Can you work these out from the model? Positions are in its coordinate system, mm. Give positions to 0.01 mm unless a question says otherwise; leave off trailing zeros. Order: outer loops, then holes, each group sorted by start corner. A loop starts at its lowest first (then second) coordinate and runs counter-clockwise, first axis right, second up. Notation, with made-up numbers: M 9,-30.5 L 48,-30.5 A25 ccw 48,-2.5 Z; hole C 28,28 d10. An arc over 180 degrees is marked long. Use a Markdown table: item, result. Add a question column.
Autodesk Inventor part; units mm, degrees
ref_plane "YZ Plane" through (0, 0, 0) normal (1, 0, 0) x (0, 1, 0)
ref_plane "XZ Plane" through (0, 0, 0) normal (0, 1, 0) x (-1, 0, 0)
ref_plane "XY Plane" through (0, 0, 0) normal (0, 0, 1) x (1, 0, 0)
sketch "Sketch1" plane through (0, 0, 0) normal (0, 0, 1) x (1, 0, 0)
  arc A0 (-142.7162, -169.544) -> (-130.9605, -185.7243) centre (-136.8383, -177.6341) ccw
  line L0 (-17.6981, -103.4344) -> (-130.9605, -185.7243)
  line L1 (46.5951, -32.0012) -> (-142.7162, -169.544)
  line L2 (-17.6981, -103.4344) -> (58.3508, -48.1816)
  arc A1 (58.3508, -48.1816) -> (46.5951, -32.0012) centre (52.473, -40.0914) ccw
  circle A2 centre (52.473, -40.0914) radius 4
  circle A3 centre (-136.8383, -177.6341) radius 6
  point P0 (0, 0)
  point P1 (0, 0)
  dimension "d0" = 8
  dimension "d3" = 12
extrude "Extrusion1" add sketch "Sketch1" along normal mid plane 24
properties part number "Second part of arm of gripper"
1. I need wall thicknesses on L1, parallel to Y at x = -131.5, z = -9.25; L2, parallel to Y at x = -93.5, z = 4; L3, parallel to Y at x = 43.5, z = 10. Which ranges of each line are inside material? Lowest first, please. Write a range as [from, to].
2. If we section it at C-C, the plane x = -89: List the corners of the cut face in (y, z) for me.
3. If we section it at B-B, the plane y = -130: List the corners of the cut face in (x, z) for me.
4. If we section it at A-A, the plane z = 5.5: List the corners of the cut face in (x, y) for me.
5. We'd pull the mould along Y, two halves only. Please class faces 1 (the face through (-43, -108, -12)), 2 (the face through (48.477, -40.267, -0.168)), 3 (the face through (-131.296, -175.336, -0.168)), 4 (the face through (-144.797, -183.688, -0.168)): +Y half, -Y half, draft (parallel to the pull), parting line (faces both ways), or undercut.
6. Will these pins go through, and if not, where does the flat tip stop? pin 1 (1.5 mm diameter, centred on y = -123, z = 3.5, fed in from +X); pin 2 (13 mm diameter, centred on x = 52.47, y = -40.09, fed in from +Z); pin 3 (1 mm diameter, centred on x = -25, z = 3, fed in from -Y); pin 4 (2 mm diameter, centred on y = -130, z = -6.5, fed in from +X).
Geometry results:
| question | item | result |
|---|---|---|
| 1 | L1 | y = [-186.09, -180.37], [-174.9, -161.39] |
| 1 | L2 | y = [-158.51, -133.79] |
| 1 | L3 | y = [-58.97, -34.25] |
| 2 | outline | M -155.24,-12 L -130.52,-12 L -130.52,12 L -155.24,12 Z |
| 3 | outline | M -88.29,-12 L -54.26,-12 L -54.26,12 L -88.29,12 Z |
| 4 | outline | M -142.72,-169.54 A10 ccw -130.96,-185.72 L -17.7,-103.43 L 58.35,-48.18 A10 ccw 46.6,-32 Z; hole C -136.84,-177.63 d12; hole C 52.47,-40.09 d8 |
| 5 | face 1 | draft |
| 5 | face 2 | undercut |
| 5 | face 3 | undercut |
| 5 | face 4 | parting line |
| 6 | pin 1 | stops at x = -43.6 |
| 6 | pin 2 | stops at z = 12 |
| 6 | pin 3 | stops at y = -109.1 |
| 6 | pin 4 | stops at x = -52.89 |
